For this review, take the finished solid that the model builds, in its own axes (mm). Face numbers are marked on the shaded views. A direction names the side the tool comes from. Coordinates: 2 decimals unless noted, no trailing zeros. Write each loop counter-clockwise with the first axis right and the second up, starting at its lowest first coordinate (ties: lowest second). Pieces come first, ordered by that corner, then holes.
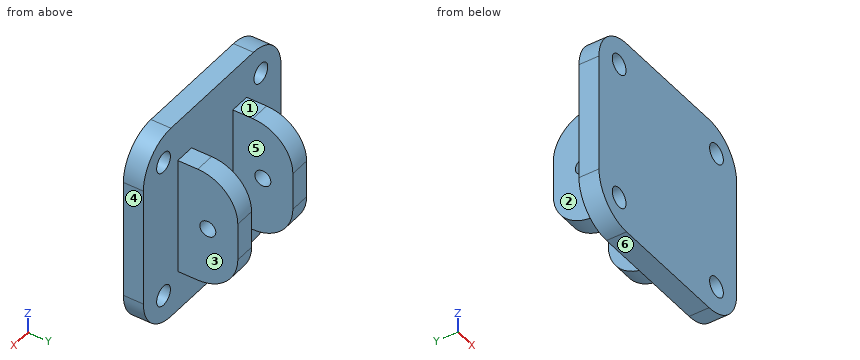
```python
from build123d import *

# Parameters (mm, degrees)
SKETCH1_W           = 50
SKETCH1_H           = 50
SKETCH1_R           = 2.5
BOSS_EXTRUDE1_DEPTH = 5
SKETCH2_W           = 5
SKETCH2_H           = 29.468657126
BOSS_EXTRUDE2_DEPTH = 15
SKETCH3_R           = 2
CUT_EXTRUDE1_DEPTH  = 50.307707308
FILLET1_R           = 10
FILLET2_R           = 10


with BuildPart() as part:
    # Sketch1 → Boss-Extrude1 (new body)
    with BuildSketch(Plane(origin=(0, 0, 0), x_dir=(1, 0, 0), z_dir=(0, 1, 0))):
        Rectangle(SKETCH1_W, SKETCH1_H)
        with Locations(Location((-17.68, 17.68, 0), (0, 0, 270))):
            Circle(SKETCH1_R, mode=Mode.SUBTRACT)
        with Locations(Location((17.68, 17.68, 0), (0, 0, 270))):
            Circle(SKETCH1_R, mode=Mode.SUBTRACT)
        with Locations(Location((17.68, -17.68, 0), (0, 0, 90))):
            Circle(SKETCH1_R, mode=Mode.SUBTRACT)
        with Locations(Location((-17.68, -17.68, 0), (0, 0, 90))):
            Circle(SKETCH1_R, mode=Mode.SUBTRACT)
    extrude(amount=BOSS_EXTRUDE1_DEPTH)

    # Sketch2 → Boss-Extrude2 (add)
    with BuildSketch(Plane(origin=(0, 5, 0), x_dir=(1, 0, 0), z_dir=(0, 1, 0))):
        with Locations((-10, 0)):
            Rectangle(SKETCH2_W, SKETCH2_H)
        with Locations((10, 0)):
            Rectangle(SKETCH2_W, SKETCH2_H)
    extrude(amount=BOSS_EXTRUDE2_DEPTH)

    # Sketch3 → Cut-Extrude1 (cut, through all)
    with BuildSketch(Plane(origin=(12.5, 0, 0), x_dir=(0, 0, -1), z_dir=(1, 0, 0))):
        with Locations((0, 12.5)):
            Circle(SKETCH3_R)
    extrude(amount=-CUT_EXTRUDE1_DEPTH, mode=Mode.SUBTRACT)

    # Fillet1
    fillet1_edges = [part.edges().sort_by_distance(p)[0] for p in [
        (-10, 20, -14.734328563),
        (-10, 20, 14.734328563),
        (10, 20, -14.734328563),
        (10, 20, 14.734328563),
    ]]
    fillet(fillet1_edges, radius=FILLET1_R)

    # Fillet2
    fillet2_edges = [part.edges().sort_by_distance(p)[0] for p in [
        (25, 2.5, 25),
        (-25, 2.5, 25),
        (-25, 2.5, -25),
        (25, 2.5, -25),
    ]]
    fillet(fillet2_edges, radius=FILLET2_R)


solid = part.part
```
1) Consider section D-D (z = -3). Give the boundary of the cut face in (x, y).
2) Consider section A-A (y = 7.25). Give the boundary of the cut face in (x, z).
3) Clearance check with flat-ended pins moving along their axes: P1, Ø1.5, axis at x = -10.5, y = 6.5, coming from the -Z side; P2, Ø4.5, axis at y = 13.5, z = 6, coming from the -X side; P3, Ø4, axis at x = 17.68, z = 17.68, coming from the -Y side; P4, Ø12, axis at y = 13.5, z = 3.5, coming from the +X side. State where each tip first meets the part, or that it passes through.
4) Tool access review of the marked faces 1, 2 and 3: name each direction out of +Z, -Z, +X, -X, +Y, -Y from which nothing blocks a thin tool from reaching the whole face with its end or side.
5) For L1, parallel to X at y = 16, z = 1; L2, parallel to X at y = 1.25, z = -18; L3, parallel to X at y = 3.1, z = 17.68, list the stretches that pass through material, from the lowest coordinate up.
6) Consider section C-C (x = 10). Give the boundary of the cut face in (y, z), then the cut area to 3 significant figures.
7) The part is to be moulded in two halves that separate along X. For the marked faces 4, 5 and 6, say which applies: pulls with the +X half, pulls with the -X half, needs draft (parallel to the pull), parting line crosses it, or undercut.
8) Consider section B-B (y = 13.5). Give the boundary of the cut face in (x, z).
Results:
1. outline: (-25, 0) - (25, 0) - (25, 5) - (12.5, 5) - (12.5, 20) - (7.5, 20) - (7.5, 5) - (-7.5, 5) - (-7.5, 20) - (-12.5, 20) - (-12.5, 5) - (-25, 5) - close
2. outline: (-12.5, -14.73) - (-7.5, -14.73) - (-7.5, 14.73) - (-12.5, 14.73) - close; (7.5, -14.73) - (12.5, -14.73) - (12.5, 14.73) - (7.5, 14.73) - close
3. P1: stops at z = -14.73
3. P2: stops at x = -12.5
3. P3: passes through
3. P4: stops at x = 12.5
4. face 1: +Z, +X, -X, +Y
4. face 2: +Z, -Z, -X, +Y
4. face 3: +Z, -Z, +X, +Y
5. L1: x = -12.5 to -7.5, 7.5 to 12.5
5. L2: x = -24.54 to -20.16, -15.2 to 15.2, 20.16 to 24.54
5. L3: x = -24.63 to -20.18, -15.18 to 15.18, 20.18 to 24.63
6. outline: (0, -25) - (5, -25) - (5, -14.73) - (10, -14.73) arc R10 ccw to (20, -4.73) - (20, 4.73) arc R10 ccw to (10, 14.73) - (5, 14.73) - (5, 25) - (0, 25) - close; hole circle Ø4 at (12.5, 0)
6. area: 637 mm2
7. face 4: pulls with the +X half
7. face 5: undercut
7. face 6: needs draft
8. outline: (-12.5, -14.1) - (-7.5, -14.1) - (-7.5, -1.73) - (-12.5, -1.73) - close; (-12.5, 1.73) - (-7.5, 1.73) - (-7.5, 14.1) - (-12.5, 14.1) - close; (7.5, -14.1) - (12.5, -14.1) - (12.5, -1.73) - (7.5, -1.73) - close; (7.5, 1.73) - (12.5, 1.73) - (12.5, 14.1) - (7.5, 14.1) - close
